Can you work these out from the drawing? Everything is in mm from the part's minimum corner. Coordinates: 2 decimals unless noted, no trailing zeros. Loops run counter-clockwise (first coordinate to the right, second up) from the corner with the lowest first, then second, coordinate; pieces in that order, holes last. Notation, with made-up numbers: (18.5, 70.25) - (70.5, 70.25) arc R27 ccw to (70.5, 109.25) - close; hole circle Ø3 at (68, 37.5). An arc over 180 degrees is marked (long way). One line per question, with ' | ' between items. Start each with the question number.
1. I want a section at A-A, the plane z = 1.25. Write out the boundary of the cut face in (x, y) (1 decimal).
2. Please list where these lines run through material, in increasing order: L1, parallel to Z at x = 4, y = 2.25; L2, parallel to X at y = 7, z = 3.5; L3, parallel to X at y = 5.75, z = 9.75 (1 decimal). Write a range as [from, to].
3. I want a section at C-C, the plane z = 8.75. Write out the boundary of the cut face in (x, y) (1 decimal), then the cut area to 3 significant figures.
4. I'm going to push flat-ended pins straight in: P1, Ø1, axis at x = 9, z = 7, coming from the -Y side; P2, Ø5, axis at y = 2.5, z = 8, coming from the -X side; P3, Ø4, axis at x = 10.5, y = 11.5, coming from the -Z side. Where does each tip first touch, or does it pass through?
5. I want a section at B-B, the plane y = 13.75. Write out the boundary of the cut face in (x, z) (1 decimal), then the cut area to 3 significant figures.
6. We'd pull the mould along Y, two halves only. Please class the marked faces 1, 2 and 3: pulls with the +Y half, pulls with the -Y half, needs draft (parallel to the pull), parting line crosses it, or undercut.
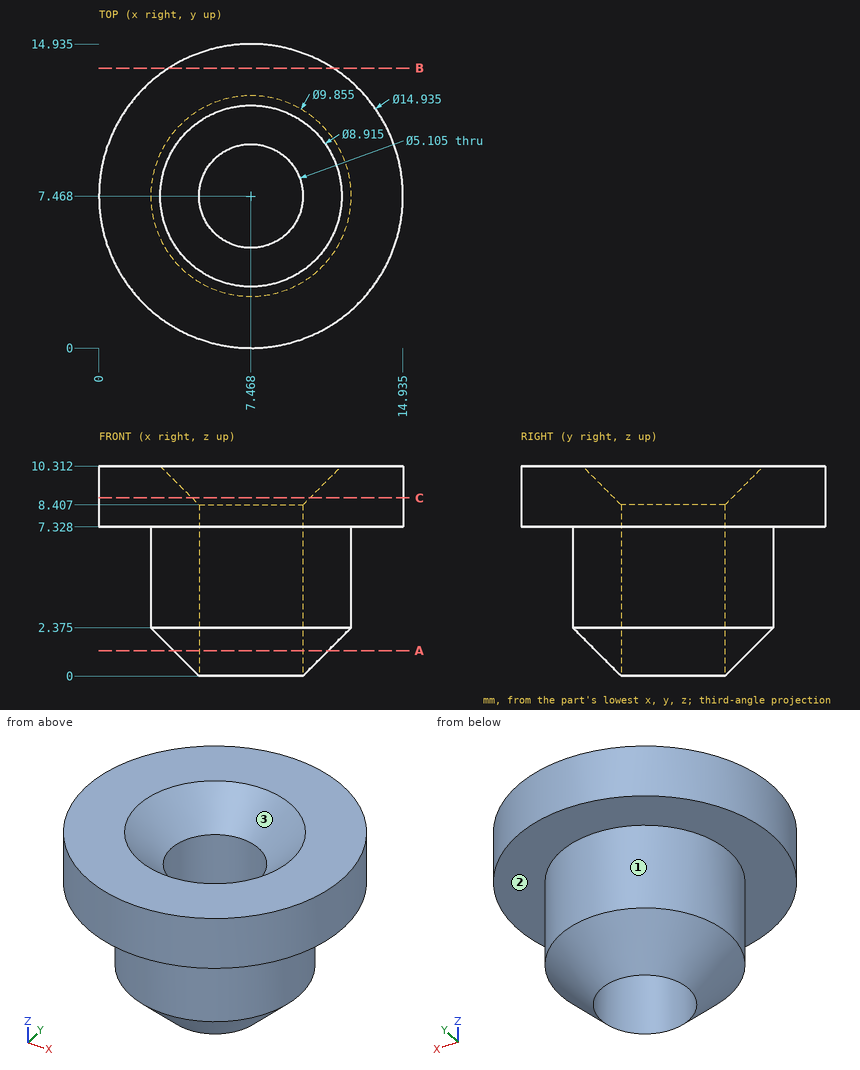
Results are:
1) outline: circle Ø7.6 at (7.5, 7.5); hole circle Ø5.1 at (7.5, 7.5)
2) L1: z = [7.33, 10.31] | L2: x = [2.56, 4.96], [9.98, 12.37] | L3: x = [0.2, 4], [11, 14.7]
3) outline: circle Ø14.9 at (7.5, 7.5); hole circle Ø5.8 at (7.5, 7.5) | area: 149 mm2
4) P1: stops at y = 0.09 | P2: stops at x = 0.42 | P3: stops at z = 0.49
5) outline: (3.4, 7.3) - (11.5, 7.3) - (11.5, 10.3) - (3.4, 10.3) - close | area: 24.1 mm2
6) face 1: parting line crosses it | face 2: needs draft | face 3: undercut
